Input: dimensioned drawing with shaded views. Units: mm. Origin: part minimum x, y, z. A direction names the side the tool comes from. Round coordinates to 2 decimals unless told otherwise and drop trailing zeros. Write each loop counter-clockwise with the first axis right and the second up, starting at its lowest first coordinate (ties: lowest second). Pieces come first, ordered by that corner, then holes. Notation, with made-up numbers: (23, 32) - (53, 32) arc R25 ccw to (53, 63) - close; hole circle Ø10 at (36.25, 20.25). An arc over 180 degrees is marked (long way). Use one line per item in the form item = value.
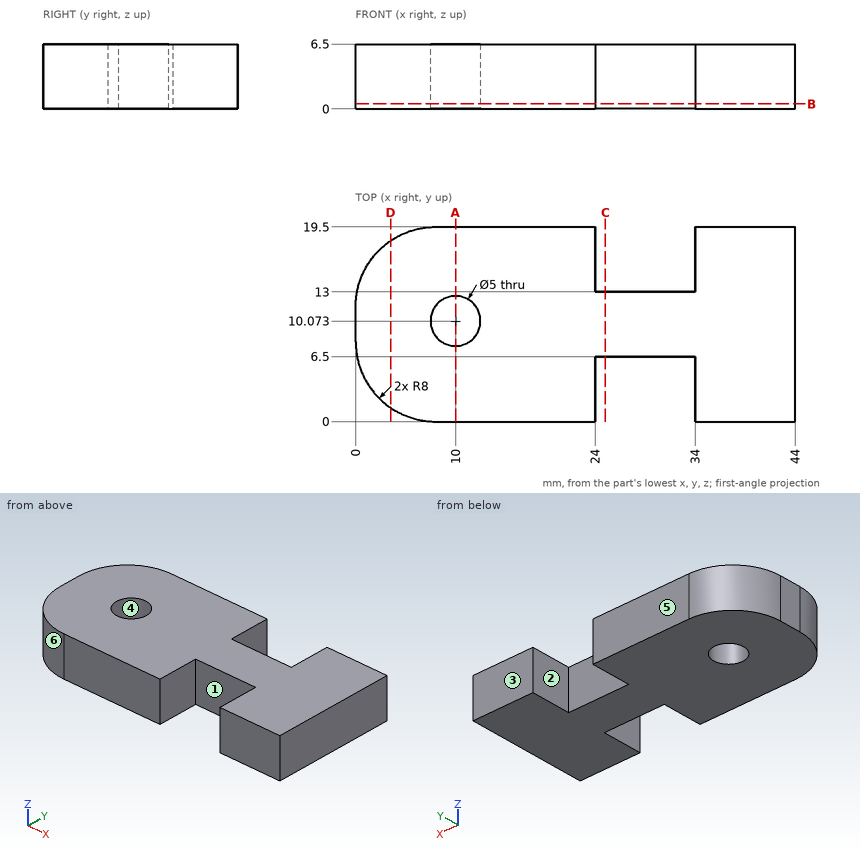
(1) Cut plane C-C on x = 25. Output: boundary loops of the cut face in (y, z).
Derived:
outline = (6.5, 0) - (13, 0) - (13, 6.5) - (6.5, 6.5) - close
(2) Access query for the marked faces 1, 2 and 3. Directions: +Z, -Z, +X, -X, +Y, -Y. A direction counts if a zero-diameter tool reaches every point of the face in a straight line with its end or side. Return the directions, or none.
Derived:
face_1 = +Z, -Z, -Y
face_2 = +Z, -Z, +Y
face_3 = +Z, -Z, +X, -X, +Y
(3) Cut plane D-D on x = 3.5. Output: boundary loops of the cut face in (y, z), then the cut area to 3 significant figures.
Derived:
outline = (1.39, 0) - (18.11, 0) - (18.11, 6.5) - (1.39, 6.5) - close
area = 109 mm^2
(4) Material intervals for L1, parallel to Y at x = 10, z = 4.5; L2, parallel to Y at x = 10.5, z = 1.5; L3, parallel to Y at x = 31, z = 5.75, sorted ascending.
Derived:
L1 = 0 to 7.57, 12.57 to 19.5
L2 = 0 to 7.62, 12.52 to 19.5
L3 = 6.5 to 13
(5) Draft query along Y for the marked faces 4, 5 and 6. Return one class per face: released by +Y, released by -Y, zero draft, split by the parting line, or undercut.
Derived:
face_4 = undercut
face_5 = released by +Y
face_6 = released by -Y
(6) First-contact query: pin 1 Ø8 at (x, y) = (10, 10.07) entering from -Z; pin 2 Ø1.5 at (y, z) = (14.5, 4.5) entering from -X; pin 3 Ø2 at (x, z) = (29, 2) entering from +Y; pin 4 Ø2 at (y, z) = (4.5, 3.5) entering from -X. Flat tips, straight axial feed; report the tip coordinate or a pass-through.
Derived:
pin_1 = 0
pin_2 = 0.32
pin_3 = 13
pin_4 = 0.4
(7) Cut plane B-B on z = 0.5. Output: boundary loops of the cut face in (x, y), then the cut area to 3 significant figures.
Derived:
outline = (0, 8) arc R8 ccw to (8, 0) - (24, 0) - (24, 6.5) - (34, 6.5) - (34, 0) - (44, 0) - (44, 19.5) - (34, 19.5) - (34, 13) - (24, 13) - (24, 19.5) - (8, 19.5) arc R8 ccw to (0, 11.5) - close; hole circle Ø5 at (10, 10.07)
area = 681 mm^2
(8) Cut plane A-A on x = 10. Output: boundary loops of the cut face in (y, z).
Derived:
outline = (0, 0) - (7.57, 0) - (7.57, 6.5) - (0, 6.5) - close; (12.57, 0) - (19.5, 0) - (19.5, 6.5) - (12.57, 6.5) - close
